Here's the drawing with two shaded views (mm, measured from the low corner). I have some questions. Round coordinates to 2 decimals unless told otherwise and drop trailing zeros. Order: outer loops, then holes, each group sorted by start corner. A loop starts at its lowest first (then second) coordinate and runs counter-clockwise, first axis right, second up. Notation, with made-up numbers: (88.25, 48.5) -> (133.25, 48.5) arc R31 cw to (133.25, 79.5) -> close; hole circle Ø8 at (-0.5, -12.75). An arc over 180 degrees is marked (long way). Use a Markdown table: item, result. Add a question column.
Q1. I need wall thicknesses on line 1 along Z through (x, y) = (2.5, 16); line 2 along Z through (x, y) = (2.55, 70); line 3 along Y through (x, z) = (2.7, 41). Which ranges of each line are inside material? Lowest first, please. Write a range as [from, to].
Q2. If we section it at C-C on y = 160.5: List the corners of the cut face in (x, z) for me.
Q3. If we section it at B-B on z = 26: List the corners of the cut face in (x, y) for me.
Q4. If we section it at A-A on x = 0.95: Give the number of separate pieces and of enclosed holes in the cut face, plus the area to 3 significant figures.
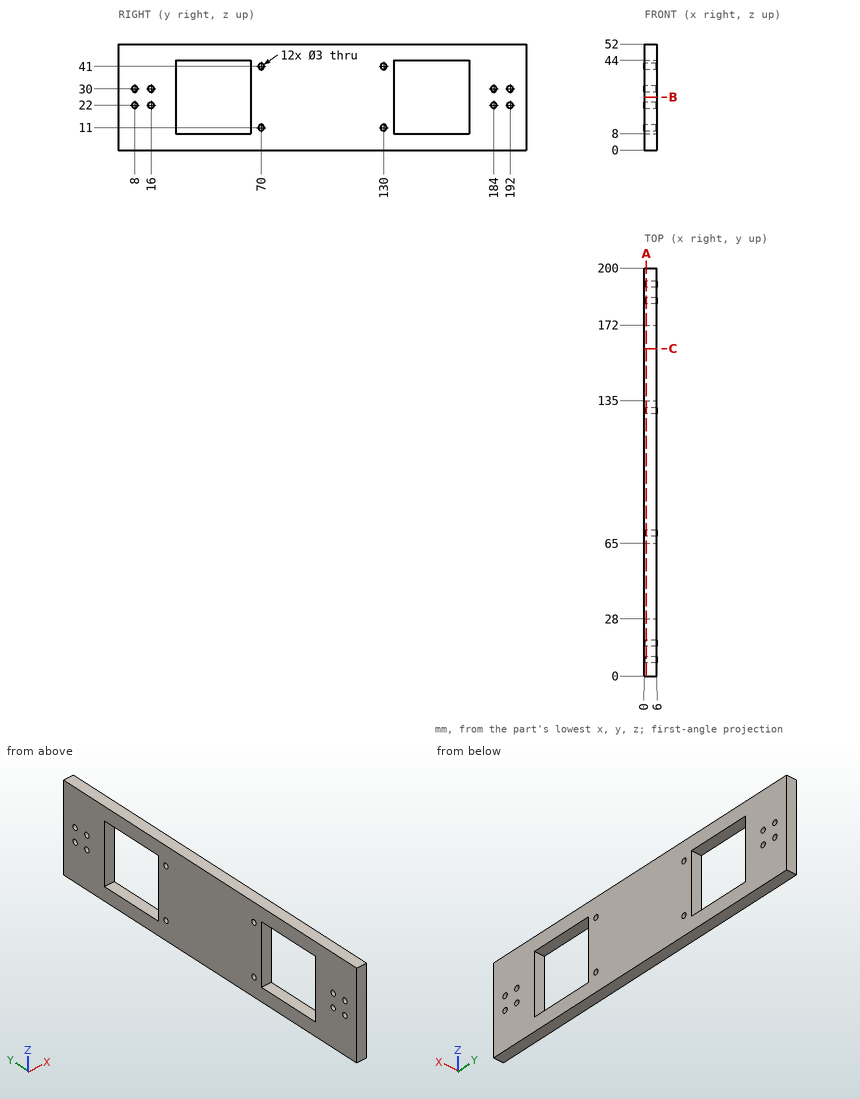
Answer below:
| question | item | result |
|---|---|---|
| 1 | line 1 | [0, 20.5], [23.5, 28.5], [31.5, 52] |
| 1 | line 2 | [0, 9.5], [12.5, 39.5], [42.5, 52] |
| 1 | line 3 | [0, 28], [65, 68.5], [71.5, 128.5], [131.5, 135], [172, 200] |
| 2 | outline | (0, 0) -> (6, 0) -> (6, 8) -> (0, 8) -> close; (0, 44) -> (6, 44) -> (6, 52) -> (0, 52) -> close |
| 3 | outline | (0, 0) -> (6, 0) -> (6, 28) -> (0, 28) -> close; (0, 65) -> (6, 65) -> (6, 135) -> (0, 135) -> close; (0, 172) -> (6, 172) -> (6, 200) -> (0, 200) -> close |
| 4 | separate pieces | 1 |
| 4 | enclosed holes | 14 |
| 4 | area | 7,650 mm² |
